from build123d import *

# Parameters (mm, degrees)
SKETCH1_W           = 45
SKETCH1_H           = 28
BOSS_EXTRUDE1_DEPTH = 13.97
BOSS_EXTRUDE2_DEPTH = 3.81
SKETCH4_R           = 1
SKETCH4_R_2         = 2
BOSS_EXTRUDE3_DEPTH = 10


with BuildPart() as part:
    # Sketch1 → Boss-Extrude1 (new body)
    with BuildSketch(Plane.XY):
        Rectangle(SKETCH1_W, SKETCH1_H)
    extrude(amount=BOSS_EXTRUDE1_DEPTH)

    # Sketch3 → Boss-Extrude2 (add)
    with BuildSketch(Plane(origin=(0, 0, 0), x_dir=(-1, 0, 0), z_dir=(0, 0, -1))):
        with BuildLine():
            Line((-22.5, 6.35), (-29.854033425, 2.72651182))
            ThreePointArc((-29.854033425, 2.72651182), (-30.12, 2.164544965), (-29.633042142, 1.778))
            Line((-29.633042142, 1.778), (-25.278, 1.778))
            ThreePointArc((-25.278, 1.778), (-23.5, 0), (-25.278, -1.778))
            Line((-25.278, -1.778), (-29.633042142, -1.778))
            ThreePointArc((-29.633042142, -1.778), (-30.12, -2.164544965), (-29.854033425, -2.72651182))
            Line((-29.854033425, -2.72651182), (-22.5, -6.35))
            Line((-22.5, -6.35), (-22.5, 6.35))
        make_face()
    boss_extrude2 = extrude(amount=-BOSS_EXTRUDE2_DEPTH)

    # Mirror8: Boss-Extrude2 across plane
    add(boss_extrude2.mirror(Plane(origin=(0, 0, 0), x_dir=(0, 0, 1), z_dir=(1, 0, 0))))

    # Sketch4 → Boss-Extrude3 (add)
    with BuildSketch(Plane.XZ.offset(14)):
        with Locations(Location((-21, 10.97, 0), (0, 0, 90))):
            Circle(SKETCH4_R)
        with Locations(Location((-18.9, 10.97, 0), (0, 0, 90))):
            Circle(SKETCH4_R)
        with Locations(Location((19.5, 10.97, 0), (0, 0, 90))):
            Circle(SKETCH4_R_2)
    extrude(amount=BOSS_EXTRUDE3_DEPTH)


solid = part.part
Part model, mm, in its own coordinate system. A direction names the side the tool comes from. Give positions to 0.01 mm unless a question says otherwise; leave off trailing zeros. Loops run counter-clockwise (first coordinate to the right, second up) from the corner with the lowest first, then second, coordinate; pieces in that order, holes last. Notation, with made-up numbers: (-21, 87) -> (2, 87) arc R24 ccw to (2, 97) -> close; hole circle Ø2 at (75, 25.5). An arc over 180 degrees is marked (long way). Write each question's results on one line, items separated by ' | '. Start each with the question number.
Q1. Which spindle directions (+Z, -Z, +X, -X, +Y, -Y) get a long thin tool onto all of the face, cutting with end or side? Do faces 1 (the face through (-27, -1.778, 2)), 2 (the face through (-23.8, -1.3, 3.81)), 3 (the face through (-19, -24, 11)), 4 (the face through (27, 1.778, 2)), 5 (the face through (-20.11, -18.93, 11.43)). Say none if no direction does.
Q2. Band-saw the part on C-C on y = -21. List the corners of the cut face in (x, z).
Q3. Pin check, flat tips, straight feed: P1, Ø1, axis at y = -11.5, z = 5, coming from the -X side; P2, Ø6, axis at x = 28, y = 0.5, coming from the +Z side; P3, Ø4, axis at x = -28.5, z = 1.5, coming from the -Y side. Stop position of each tip, or through.
Q4. Band-saw the part on D-D on y = 0. List the corners of the cut face in (x, z), plus the area to 3 significant figures.
Q5. Band-saw the part on A-A on x = -18.9. List the corners of the cut face in (y, z).
Q6. Wall check: L1, parallel to Y at x = -9, z = 4.75; L2, parallel to X at y = 3, z = 12.5; L3, parallel to X at y = -21, z = 10.5. Give the ranges that are in metal, low to high.
Q7. Band-saw the part on B-B on z = 10.97. List the corners of the cut face in (x, y), plus the area to 3 significant figures.
Q8. Pull direction X, two halves, no side cores. Call faces 6 (the face through (-19.74, -18.93, 11.51)), 7 (the face through (22.5, 0, 8)), 8 (the face through (0, 0, 13.97)): +X half, -X half, draft (parallel to the pull), parting line (faces both ways), or undercut.
Results are:
1) face 1: +Z, -Z, -X | face 2: +Z, -X, +Y, -Y | face 3: +Z, -Z, +X, -X, -Y | face 4: +Z, -Z, +X | face 5: -Y
2) outline: circle Ø2 at (-21, 10.97); circle Ø2 at (-18.9, 10.97); circle Ø4 at (19.5, 10.97)
3) P1: stops at x = -22.5 | P2: stops at z = 3.81 | P3: stops at y = -4.38
4) outline: (-23.5, 0) -> (23.5, 0) -> (23.5, 3.81) -> (22.5, 3.81) -> (22.5, 13.97) -> (-22.5, 13.97) -> (-22.5, 3.81) -> (-23.5, 3.81) -> close | area: 636 mm²
5) outline: (-24, 9.97) -> (-14, 9.97) -> (-14, 0) -> (14, 0) -> (14, 13.97) -> (-14, 13.97) -> (-14, 11.97) -> (-24, 11.97) -> close
6) L1: y = -14 to 14 | L2: x = -22.5 to 22.5 | L3: x = -21.88 to -20.12, -19.78 to -18.02, 17.56 to 21.44
7) outline: (-22.5, -14) -> (-22, -14) -> (-22, -24) -> (-20, -24) -> (-20, -14) -> (-19.9, -14) -> (-19.9, -24) -> (-17.9, -24) -> (-17.9, -14) -> (17.5, -14) -> (17.5, -24) -> (21.5, -24) -> (21.5, -14) -> (22.5, -14) -> (22.5, 14) -> (-22.5, 14) -> close | area: 1,340 mm²
8) face 6: undercut | face 7: +X half | face 8: draft
